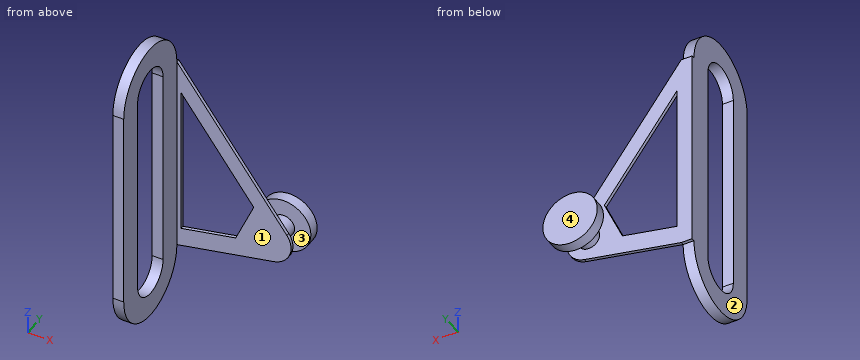
from build123d import *

# Parameters (mm, degrees)
BOSS_EXTRUDE1_DEPTH = 10
BOSS_EXTRUDE2_DEPTH = 3
SKETCH3_R           = 10
BOSS_EXTRUDE3_DEPTH = 20
CUT_EXTRUDE1_DEPTH  = 11
CUT_EXTRUDE2_DEPTH  = 89
SKETCH6_R           = 25
BOSS_EXTRUDE4_DEPTH = 10


with BuildPart() as part:
    # Sketch1 → Boss-Extrude1 (new body)
    with BuildSketch(Plane(origin=(0, 0, 0), x_dir=(0, -1, 0), z_dir=(-1, 0, 0))):
        with BuildLine():
            Line((-42.5, 186), (-42.5, 0))
            ThreePointArc((-42.5, 0), (0, -42.5), (42.5, 0))
            Line((42.5, 0), (42.5, 186))
            ThreePointArc((42.5, 186), (0, 228.5), (-42.5, 186))
        make_face()
    extrude(amount=-BOSS_EXTRUDE1_DEPTH)

    # Sketch2 → Boss-Extrude2 (add)
    with BuildSketch(Plane(origin=(0, 42.5, 0), x_dir=(-1, 0, 0), z_dir=(0, 1, 0))):
        with BuildLine():
            Line((-10, 0), (-98.944350751, 17.892804965))
            ThreePointArc((-98.944350751, 17.892804965), (-113.663663971, 30.311978912), (-111.07737178, 49.396138729))
            Line((-111.07737178, 49.396138729), (-10, 186))
            Line((-10, 186), (0, 186))
            Line((0, 186), (0, 0))
            Line((0, 0), (-10, 0))
        make_face()
    extrude(amount=BOSS_EXTRUDE2_DEPTH)

    # Sketch3 → Boss-Extrude3 (add)
    with BuildSketch(Plane(origin=(0, 45.5, 0), x_dir=(-1, 0, 0), z_dir=(0, 1, 0))):
        with Locations((-95, 37.5)):
            Circle(SKETCH3_R)
    extrude(amount=BOSS_EXTRUDE3_DEPTH)

    # Sketch4 → Cut-Extrude1 (cut, through all)
    with BuildSketch(Plane(origin=(10, 0, 0), x_dir=(0, 0, -1), z_dir=(1, 0, 0))):
        with BuildLine():
            Line((0, 20.390002673), (-186, 20.390002673))
            ThreePointArc((-186, 20.390002673), (-206.390002673, 0), (-186, -20.390002673))
            Line((-186, -20.390002673), (0, -20.390002673))
            ThreePointArc((0, -20.390002673), (20.390002673, 0), (0, 20.390002673))
        make_face()
    extrude(amount=-CUT_EXTRUDE1_DEPTH, mode=Mode.SUBTRACT)

    # Sketch5 → Cut-Extrude2 (cut, through all)
    with BuildSketch(Plane(origin=(0, 45.5, 0), x_dir=(-1, 0, 0), z_dir=(0, 1, 0))):
        Polygon((-64.102931729, 28.152292708), (-13.715935026, 18.016014269), (-13.715935026, 156.359237723), (-80.693023557, 65.841164794), align=None)
    extrude(amount=-CUT_EXTRUDE2_DEPTH, mode=Mode.SUBTRACT)

    # Sketch6 → Boss-Extrude4 (add)
    with BuildSketch(Plane(origin=(0, 65.5, 0), x_dir=(1, 0, 0), z_dir=(0, 1, 0))):
        with Locations((95, -37.5)):
            Circle(SKETCH6_R)
    extrude(amount=BOSS_EXTRUDE4_DEPTH)


solid = part.part
Input: part model. Units: mm. Frame: model coordinates. Face numbers are marked on the shaded views. Give positions to 0.01 mm unless a question says otherwise; leave off trailing zeros. Write each loop counter-clockwise with the first axis right and the second up, starting at its lowest first coordinate (ties: lowest second). Pieces come first, ordered by that corner, then holes.
Q1. Section A-A, the plane y = 0. Output: boundary loops of the cut face in (x, z), plus the area to 3 significant figures.
Q2. Section D-D, the plane x = 93.5. Output: boundary loops of the cut face in (y, z), plus the area to 3 significant figures.
Q3. Material intervals for probe 1 along Y at (x, z) = (77, 24); probe 2 along X at (y, z) = (40, 154); probe 3 along Y at (x, z) = (42, 17.5), sorted ascending.
Q4. Section B-B, the plane z = 162. Output: boundary loops of the cut face in (x, y).
Q5. Pull-direction query (Y, two-part tool) for the marked faces 1, 2, 3 and 4; classes: pulls with the +Y half, pulls with the -Y half, needs draft (parallel to the pull), parting line crosses it, or undercut.
Q6. Section C-C, the plane z = 37.5. Output: boundary loops of the cut face in (x, y).
Q7. First-contact query: P1, Ø15, axis at x = 101.5, z = 33.5, coming from the -Y side; P2, Ø10, axis at x = 65.5, y = 41, coming from the +Z side; P3, Ø4, axis at x = 24, y = 48, coming from the +Z side; P4, Ø3.5, axis at y = 43.5, z = 92, coming from the +X side. Flat tips, straight axial feed; report the tip coordinate or a pass-through.
Filled in:
1. outline: (0, -42.5) - (10, -42.5) - (10, -20.39) - (0, -20.39) - close; (0, 206.39) - (10, 206.39) - (10, 228.5) - (0, 228.5) - close
1. area: 442 mm2
2. outline: (42.5, 16.8) - (45.5, 16.8) - (45.5, 27.61) - (65.5, 27.61) - (65.5, 12.55) - (75.5, 12.55) - (75.5, 62.45) - (65.5, 62.45) - (65.5, 47.39) - (45.5, 47.39) - (45.5, 73.15) - (42.5, 73.15) - close
2. area: 1,060 mm2
3. probe 1: y = 42.5 to 45.5, 65.5 to 75.5
3. probe 2: x = 0 to 10
3. probe 3: y = 42.5 to 45.5
4. outline: (0, -42.5) - (10, -42.5) - (10, -20.39) - (0, -20.39) - close; (0, 20.39) - (10, 20.39) - (10, 42.5) - (27.76, 42.5) - (27.76, 45.5) - (0, 45.5) - close
5. face 1: pulls with the -Y half
5. face 2: needs draft
5. face 3: undercut
5. face 4: pulls with the +Y half
6. outline: (0, -42.5) - (10, -42.5) - (10, -20.39) - (0, -20.39) - close; (0, 20.39) - (10, 20.39) - (10, 42.5) - (13.72, 42.5) - (13.72, 45.5) - (0, 45.5) - close; (68.22, 42.5) - (115, 42.5) - (115, 45.5) - (105, 45.5) - (105, 65.5) - (120, 65.5) - (120, 75.5) - (70, 75.5) - (70, 65.5) - (85, 65.5) - (85, 45.5) - (68.22, 45.5) - close
7. P1: stops at y = 42.5
7. P2: stops at z = 117.44
7. P3: passes through
7. P4: stops at x = 80.85
